The listing builds one solid part. Answer for the finished solid, in the listing's coordinates (mm). Give positions to 0.01 mm unless a question says otherwise; leave off trailing zeros. Loops run counter-clockwise (first coordinate to the right, second up) from the corner with the lowest first, then second, coordinate; pieces in that order, holes last. Notation, with made-up numbers: M 6,-30.75 L 27,-30.75 A15 ccw 27,-18.75 Z; hole C 43,7.25 d5. An arc over 180 degrees is marked long. Return JSON: item names as keys, results as strings.
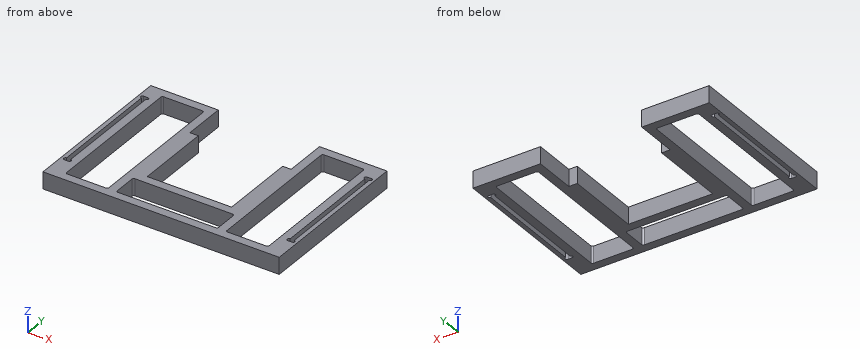
Autodesk Inventor part; units mm, degrees
ref_plane "YZ Plane" through (0, 0, 0) normal (1, 0, 0) x (0, 1, 0)
ref_plane "XZ Plane" through (0, 0, 0) normal (0, 1, 0) x (-1, 0, 0)
ref_plane "XY Plane" through (0, 0, 0) normal (0, 0, 1) x (1, 0, 0)
sketch "スケッチ1" plane through (0, 0, 0) normal (0, 0, 1) x (1, 0, 0)
  line L0 (0, 0) -> (140, 0)
  line L1 (140, 0) -> (140, 95)
  line L2 (0, 95) -> (0, 0)
  line L3 (70, 94.6562) -> (70, 0) construction
  line L4 (95, 70) -> (95, 25)
  line L5 (95, 25) -> (45, 25)
  line L6 (45, 25) -> (45, 70)
  line L7 (140, 95) -> (100, 95)
  line L8 (40, 95) -> (0, 95)
  line L9 (100, 95) -> (100, 70)
  line L10 (40, 70) -> (40, 95)
  line L11 (100, 70) -> (95, 70)
  line L12 (45, 70) -> (40, 70)
  dimension "d0" = 140
  dimension "d1" = 95
  dimension "d2" = 25
  dimension "d3" = 50
  dimension "d4" = 60
  dimension "d6" = 25
extrude "押し出し1" add sketch "スケッチ1" along normal blind 10
sketch "スケッチ2" plane through (0, 0, 10) normal (0, 0, 1) x (1, 0, 0)
  line L0 (0, 0) -> (140, 0)
  line L1 (70, 0) -> (70, 25) construction
  line L2 (95, 25) -> (45, 25)
  line L3 (135, 85) -> (137.5, 85)
  line L4 (137.5, 83) -> (137.5, 17)
  line L5 (137.5, 15) -> (135, 15)
  line L6 (135, 17) -> (135, 83)
  line L7 (140, 95) -> (100, 95)
  line L8 (140, 0) -> (140, 95)
  arc A0 (135, 85) -> (135, 83) centre (135, 84) ccw
  arc A1 (137.5, 83) -> (137.5, 85) centre (137.5, 84) ccw
  arc A2 (135, 17) -> (135, 15) centre (135, 16) ccw
  arc A3 (137.5, 15) -> (137.5, 17) centre (137.5, 16) ccw
  line L9 (5, 85) -> (2.5, 85)
  line L10 (2.5, 83) -> (2.5, 17)
  line L11 (2.5, 15) -> (5, 15)
  line L12 (5, 17) -> (5, 83)
  arc A4 (5, 83) -> (5, 85) centre (5, 84) ccw
  arc A5 (2.5, 85) -> (2.5, 83) centre (2.5, 84) ccw
  arc A6 (5, 15) -> (5, 17) centre (5, 16) ccw
  arc A7 (2.5, 17) -> (2.5, 15) centre (2.5, 16) ccw
  dimension "d9" = 15
  dimension "d10" = 10
  dimension "d11" = 2.5
  dimension "d12" = 2.5
  dimension "d16" = 2
  dimension "d17" = 1
  dimension "d18" = 2
  dimension "d19" = 1
extrude "押し出し2" cut sketch "スケッチ2" against normal through all
sketch "スケッチ3" plane through (0, 0, 10) normal (0, 0, 1) x (1, 0, 0)
  line L0 (40, 20) -> (100, 20)
  line L1 (100, 20) -> (100, 5)
  line L2 (100, 5) -> (40, 5)
  line L3 (40, 5) -> (40, 20)
  arc A0 (135, 85) -> (135, 83) centre (135, 84) ccw
  line L4 (135, 85) -> (137.5, 85)
  arc A1 (137.5, 83) -> (137.5, 85) centre (137.5, 84) ccw
  line L5 (137.5, 83) -> (137.5, 17)
  arc A2 (137.5, 15) -> (137.5, 17) centre (137.5, 16) ccw
  line L6 (137.5, 15) -> (135, 15)
  arc A3 (135, 17) -> (135, 15) centre (135, 16) ccw
  line L7 (135, 17) -> (135, 83)
  arc A4 (5, 83) -> (5, 85) centre (5, 84) ccw
  line L8 (5, 83) -> (5, 17)
  arc A5 (5, 15) -> (5, 17) centre (5, 16) ccw
  line L9 (5, 15) -> (2.5, 15)
  arc A6 (2.5, 17) -> (2.5, 15) centre (2.5, 16) ccw
  line L10 (2.5, 17) -> (2.5, 83)
  arc A7 (2.5, 85) -> (2.5, 83) centre (2.5, 84) ccw
  line L11 (2.5, 85) -> (5, 85)
  line L12 (140, 0) -> (140, 95)
  line L13 (140, 95) -> (100, 95)
  line L14 (100, 95) -> (100, 70)
  line L15 (100, 70) -> (95, 70)
  line L16 (95, 70) -> (95, 25)
  line L17 (95, 25) -> (45, 25)
  line L18 (45, 25) -> (45, 70)
  line L19 (45, 70) -> (40, 70)
  line L20 (40, 70) -> (40, 95)
  line L21 (40, 95) -> (0, 95)
  line L22 (0, 95) -> (0, 0)
  line L23 (0, 0) -> (140, 0)
  line L24 (45, 25) -> (45, 70)
  line L25 (95, 70) -> (95, 25)
  line L26 (105, 90) -> (130, 90)
  line L27 (130, 90) -> (130, 5)
  line L28 (130, 5) -> (105, 5)
  line L29 (105, 5) -> (105, 90)
  line L30 (95, 25) -> (45, 25)
  line L31 (70, 25) -> (70, 0) construction
  line L32 (35, 90) -> (10, 90)
  line L33 (10, 90) -> (10, 5)
  line L34 (10, 5) -> (35, 5)
  line L35 (35, 5) -> (35, 90)
  dimension "d20" = 5
  dimension "d21" = 5
  dimension "d22" = 5
  dimension "d23" = 5
  dimension "d24" = 10
  dimension "d25" = 5
  dimension "d26" = 5
extrude "押し出し3" cut sketch "スケッチ3" against normal through all contours L0 L1 L2 L3 | L26 L27 L28 L29 | L35 L34 L33 L32
fillet "フィレット1" radius 1 12 edges at (35, 90, 5) (10, 90, 5) (10, 5, 5) (35, 5, 5) (40, 5, 5) (40, 20, 5) (100, 5, 5) (100, 20, 5) (130, 90, 5) (105, 90, 5) (105, 5, 5) (130, 5, 5)
properties part number "waist2" material "アルミニウム 6061"
(1) Straight lines are drawn through the part: line 1 along X through (y, z) = (29.5, 3); line 2 along X through (y, z) = (87, 3.5); line 3 along X through (y, z) = (22.5, 5.5). For each, find the intervals that lie inside material, in ascending order.
Values follow:
{"line 1": "0 to 2.5, 5 to 10, 35 to 45, 95 to 105, 130 to 135, 137.5 to 140", "line 2": "0 to 10, 35 to 40, 100 to 105, 130 to 140", "line 3": "0 to 2.5, 5 to 10, 35 to 105, 130 to 135, 137.5 to 140"}
(2) The part is cut by section A-A (x = 120.5). Determine the outline of the cut face in (y, z).
Values follow:
{"outline": "M 0,0 L 5,0 L 5,10 L 0,10 Z; M 90,0 L 95,0 L 95,10 L 90,10 Z"}
(3) The part is cut by section D-D (z = 3.75). Give the number of separate pieces and of enclosed holes in the cut face, and give its area (3 significant figures).
Values follow:
{"separate pieces": "1", "enclosed holes": "5", "area": "4,040 mm²"}
(4) The part is cut by section C-C (y = 50.5). Determine the outline of the cut face in (x, z).
Values follow:
{"outline": "M 0,0 L 2.5,0 L 2.5,10 L 0,10 Z; M 5,0 L 10,0 L 10,10 L 5,10 Z; M 35,0 L 45,0 L 45,10 L 35,10 Z; M 95,0 L 105,0 L 105,10 L 95,10 Z; M 130,0 L 135,0 L 135,10 L 130,10 Z; M 137.5,0 L 140,0 L 140,10 L 137.5,10 Z"}
(5) The part is cut by section B-B (y = 75.5). Determine the outline of the cut face in (x, z).
Values follow:
{"outline": "M 0,0 L 2.5,0 L 2.5,10 L 0,10 Z; M 5,0 L 10,0 L 10,10 L 5,10 Z; M 35,0 L 40,0 L 40,10 L 35,10 Z; M 100,0 L 105,0 L 105,10 L 100,10 Z; M 130,0 L 135,0 L 135,10 L 130,10 Z; M 137.5,0 L 140,0 L 140,10 L 137.5,10 Z"}
(6) Given pin 1 (3 mm diameter, centred on x = 32.5, y = 30, fed in from +Z), flat-ended and moving along its own axis, determine where the tip first touches the part or whether it passes through.
Values follow:
{"pin 1": "through"}
